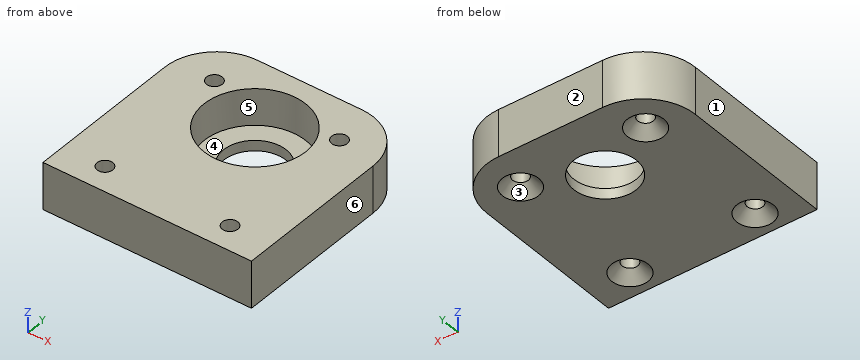
from build123d import *

# Parameters (mm, degrees)
SKETCH_W     = 40
SKETCH_H     = 40
SKETCH_R     = 6
SKETCH_R_2   = 1.5
PAD_DEPTH    = 9
SKETCH001_R  = 9.75
POCKET_DEPTH = 7
CHAMFER_SIZE = 2
FILLET_R     = 10


with BuildPart() as part:
    # Sketch → Pad (new body)
    with BuildSketch(Plane.XY):
        with Locations((0, 20)):
            Rectangle(SKETCH_W, SKETCH_H)
        with Locations((0.040094, 26.5)):
            Circle(SKETCH_R, mode=Mode.SUBTRACT)
        with Locations((-12, 32)):
            Circle(SKETCH_R_2, mode=Mode.SUBTRACT)
        with Locations((12, 32)):
            Circle(SKETCH_R_2, mode=Mode.SUBTRACT)
        with Locations((-12, 5)):
            Circle(SKETCH_R_2, mode=Mode.SUBTRACT)
        with Locations((12, 5)):
            Circle(SKETCH_R_2, mode=Mode.SUBTRACT)
    extrude(amount=PAD_DEPTH)

    # Sketch001 (on Face11 of Pad) → Pocket (cut)
    with BuildSketch(Plane.XY.offset(9)):
        with Locations((0.040094, 26.5)):
            Circle(SKETCH001_R)
    extrude(amount=-POCKET_DEPTH, mode=Mode.SUBTRACT)

    # Chamfer
    chamfer_edges = [part.edges().sort_by_distance(p)[0] for p in [
        (-13.5, 32, 0),
        (10.5, 32, 0),
        (10.5, 5, 0),
        (-13.5, 5, 0),
    ]]
    chamfer(chamfer_edges, length=CHAMFER_SIZE)

    # Fillet
    fillet_edges = [part.edges().sort_by_distance(p)[0] for p in [
        (20, 40, 4.5),
        (-20, 40, 4.5),
    ]]
    fillet(fillet_edges, radius=FILLET_R)


solid = part.part
Can you work these out from the model? Positions are in its coordinate system, mm. Face numbers are marked on the shaded views. A direction names the side the tool comes from. Give positions to 0.01 mm unless a question says otherwise; leave off trailing zeros. Loops run counter-clockwise (first coordinate to the right, second up) from the corner with the lowest first, then second, coordinate; pieces in that order, holes last. Notation, with made-up numbers: (60.5, 25.5) - (87.5, 25.5) arc R22 cw to (87.5, 59.5) - close; hole circle Ø9 at (-20, 57.25). An arc over 180 degrees is marked (long way). One line per item, written item: value.
(1) If we section it at A-A, the plane y = 26.5: List the corners of the cut face in (x, z) for me, plus the area to 4 significant figures.
Verdict:
outline: (-20, 0) - (-5.96, 0) - (-5.96, 2) - (-9.71, 2) - (-9.71, 9) - (-20, 9) - close; (6.04, 0) - (20, 0) - (20, 9) - (9.79, 9) - (9.79, 2) - (6.04, 2) - close
area: 199.5 mm^2
(2) I'm going to push flat-ended pins straight in: pin 1 (3.5 mm diameter, centred on x = 12, y = 5, fed in from +Z); pin 2 (2 mm diameter, centred on x = -11.5, y = 4.5, fed in from -Z). Where does each tip first touch, or does it pass through?
Verdict:
pin 1: z = 9
pin 2: z = 1.79
(3) On a 3-axis mill with a long thin cutter (end or side, diameter ignored), from which of +Z, -Z, +X, -X, +Y, -Y can I reach the whole of each face in a straight line? I mean the marked faces 5 and 6. Say none if no direction works.
Verdict:
face 5: +Z
face 6: +Z, -Z, +X, +Y, -Y
(4) If we section it at D-D, the plane x = 12: List the corners of the cut face in (y, z) for me.
Verdict:
outline: (0, 0) - (1.5, 0) - (3.5, 2) - (3.5, 9) - (0, 9) - close; (6.5, 2) - (8.5, 0) - (28.5, 0) - (30.5, 2) - (30.5, 9) - (6.5, 9) - close; (33.5, 2) - (35.5, 0) - (39.8, 0) - (39.8, 9) - (33.5, 9) - close
(5) I need wall thicknesses on line 1 along X through (y, z) = (4, 2.5); line 2 along X through (y, z) = (4.5, 5); line 3 along Y through (x, z) = (12.5, 2.5). Which ranges of each line are inside material? Lowest first, please.
Verdict:
line 1: -20 to -13.12, -10.88 to 10.88, 13.12 to 20
line 2: -20 to -13.41, -10.59 to 10.59, 13.41 to 20
line 3: 0 to 3.59, 6.41 to 30.59, 33.41 to 39.68
(6) If we section it at C-C, the plane y = 5: List the corners of the cut face in (x, z) for me.
Verdict:
outline: (-20, 0) - (-15.5, 0) - (-13.5, 2) - (-13.5, 9) - (-20, 9) - close; (-10.5, 2) - (-8.5, 0) - (8.5, 0) - (10.5, 2) - (10.5, 9) - (-10.5, 9) - close; (13.5, 2) - (15.5, 0) - (20, 0) - (20, 9) - (13.5, 9) - close
(7) If we mould it in two halves opening along Y, with no side actions, what happens to the marked faces 1, 2, 3 and 4? For each: released by +Y, released by -Y, zero draft, split by the parting line, or undercut.
Verdict:
face 1: zero draft
face 2: released by +Y
face 3: undercut
face 4: undercut
(8) If we section it at B-B, the plane z = 0.75: List the corners of the cut face in (x, y) for me.
Verdict:
outline: (-20, 0) - (20, 0) - (20, 30) arc R10 ccw to (10, 40) - (-10, 40) arc R10 ccw to (-20, 30) - close; hole circle Ø5.5 at (-12, 5); hole circle Ø5.5 at (-12, 32); hole circle Ø12 at (0.04, 26.5); hole circle Ø5.5 at (12, 5); hole circle Ø5.5 at (12, 32)
